Can you work these out from the model? Positions are in its coordinate system, mm. Coordinates: 2 decimals unless noted, no trailing zeros. Order: outer loops, then holes, each group sorted by start corner. A loop starts at its lowest first (then second) coordinate and runs counter-clockwise, first axis right, second up. Notation, with made-up numbers: (15, 6) -> (72, 6) arc R35 cw to (72, 45) -> close; hole circle Ø2 at (29, 71). An arc over 180 degrees is marked (long way). Answer as CSV lines item,"result".
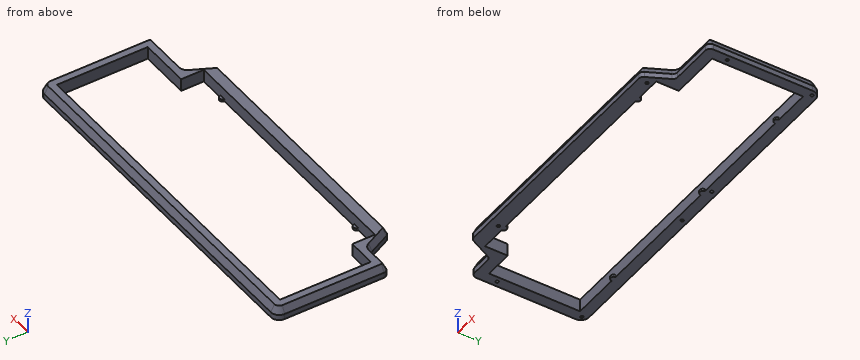
from build123d import *

# Parameters (mm, degrees)
PAD_DEPTH      = 10.6
PAD005_DEPTH   = 2
FILLET_R       = 4
FILLET014_R    = 7
CHAMFER_SIZE2  = 6
CHAMFER_SIZE   = 3
SKETCH020_R    = 1.25
HOLE007_DEPTH  = 5
HOLE007_TIPS_R = 1.25


with BuildPart() as part:
    # Sketch → Pad (new body)
    with BuildSketch(Plane.XY):
        Polygon((-152.075, 56.825), (152.075, 56.825), (152.075, -37.775), (109.7375, -37.775), (98.7125, -59.825), (-117.7625, -59.825), (-128.7875, -37.775), (-152.075, -37.775), align=None)
        Polygon((-143.075, 47.825), (143.075, 47.825), (143.075, -28.775), (100.2125, -28.775), (100.2125, -47.825), (-119.2625, -47.825), (-119.2625, -28.775), (-143.075, -28.775), align=None, mode=Mode.SUBTRACT)
    extrude(amount=PAD_DEPTH)

    # Sketch011 (on Face17 of Pad) → Pad005 (join)
    with BuildSketch(Plane(origin=(0, 0, 0), x_dir=(1, 0, 0), z_dir=(0, 0, -1))):
        with BuildLine():
            ThreePointArc((16.752533, -47.408333), (14.2875, -45.325), (11.822467, -47.408333))
            ThreePointArc((11.32946, -47.825), (11.652209, -47.706881), (11.822467, -47.408333))
            Line((11.32946, -47.825), (17.24554, -47.825))
            ThreePointArc((16.752533, -47.408333), (16.922791, -47.706881), (17.24554, -47.825))
        make_face()
        with BuildLine():
            ThreePointArc((112.002533, -47.408333), (109.5375, -45.325), (107.072467, -47.408333))
            ThreePointArc((106.57946, -47.825), (106.902209, -47.706881), (107.072467, -47.408333))
            Line((106.57946, -47.825), (112.49554, -47.825))
            ThreePointArc((112.002533, -47.408333), (112.172791, -47.706881), (112.49554, -47.825))
        make_face()
        with BuildLine():
            ThreePointArc((-97.547467, -47.408333), (-100.0125, -45.325), (-102.477533, -47.408333))
            ThreePointArc((-102.97054, -47.825), (-102.647791, -47.706881), (-102.477533, -47.408333))
            Line((-102.97054, -47.825), (-97.05446, -47.825))
            ThreePointArc((-97.547467, -47.408333), (-97.377209, -47.706881), (-97.05446, -47.825))
        make_face()
        with BuildLine():
            ThreePointArc((73.734967, 47.408333), (76.2, 45.325), (78.665033, 47.408333))
            ThreePointArc((79.15804, 47.825), (78.835291, 47.706881), (78.665033, 47.408333))
            Line((73.24196, 47.825), (79.15804, 47.825))
            ThreePointArc((73.734967, 47.408333), (73.564709, 47.706881), (73.24196, 47.825))
        make_face()
        with BuildLine():
            ThreePointArc((-97.715033, 47.408333), (-95.25, 45.325), (-92.784967, 47.408333))
            ThreePointArc((-92.29196, 47.825), (-92.614709, 47.706881), (-92.784967, 47.408333))
            Line((-98.20804, 47.825), (-92.29196, 47.825))
            ThreePointArc((-97.715033, 47.408333), (-97.885291, 47.706881), (-98.20804, 47.825))
        make_face()
    extrude(amount=-PAD005_DEPTH)

    # Fillet
    fillet_edges = [part.edges().sort_by_distance(p)[0] for p in [
        (98.7125, -59.825, 5.3),
        (109.7375, -37.775, 5.3),
        (152.075, -37.775, 5.3),
        (-117.7625, -59.825, 5.3),
        (-152.075, -37.775, 5.3),
        (-128.7875, -37.775, 5.3),
    ]]
    fillet(fillet_edges, radius=FILLET_R)

    # Fillet014
    fillet014_edges = [part.edges().sort_by_distance(p)[0] for p in [
        (152.075, 56.825, 5.3),
        (-152.075, 56.825, 5.3),
    ]]
    fillet(fillet014_edges, radius=FILLET014_R)

    # Chamfer
    chamfer_edges = [part.edges().sort_by_distance(p)[0] for p in [
        (-9.525, -59.825, 10.6),
    ]]
    chamfer_side = part.faces().sort_by_distance((148.817479, 8.025, 10.6))[0]
    chamfer(chamfer_edges, length=CHAMFER_SIZE, length2=CHAMFER_SIZE2, reference=chamfer_side)

    # Sketch020 (on Face4 of Chamfer) → Hole007 (cut)
    with BuildSketch(Plane(origin=(0, 0, 0), x_dir=(1, 0, 0), z_dir=(0, 0, -1))):
        with Locations((95.25, 52.325)):
            Circle(SKETCH020_R)
        with Locations((147.575, 19.05)):
            Circle(SKETCH020_R)
        with Locations((147.575, -52.325)):
            Circle(SKETCH020_R)
        with Locations((19.05, -52.325)):
            Circle(SKETCH020_R)
        with Locations((-19.05, -52.325)):
            Circle(SKETCH020_R)
        with Locations((-147.575, -52.325)):
            Circle(SKETCH020_R)
        with Locations((-147.575, 19.05)):
            Circle(SKETCH020_R)
        with Locations((-95.25, 52.325)):
            Circle(SKETCH020_R)
    extrude(amount=-HOLE007_DEPTH, mode=Mode.SUBTRACT)

    # Hole007 tips → Hole007 tip 1 section 0
    with BuildSketch(Plane(origin=(0, 0, 5), x_dir=(1, 0, 0), z_dir=(0, 0, -1)), mode=Mode.PRIVATE) as hole007_tip_1_s0:
        with Locations((95.25, 52.325)):
            Circle(HOLE007_TIPS_R)
    loft([hole007_tip_1_s0.sketch, Vertex(95.25, -52.325, 5.751076)], mode=Mode.SUBTRACT)

    # Hole007 tips → Hole007 tip 2 section 0
    with BuildSketch(Plane(origin=(0, 0, 5), x_dir=(1, 0, 0), z_dir=(0, 0, -1)), mode=Mode.PRIVATE) as hole007_tip_2_s0:
        with Locations((147.575, 19.05)):
            Circle(HOLE007_TIPS_R)
    loft([hole007_tip_2_s0.sketch, Vertex(147.575, -19.05, 5.751076)], mode=Mode.SUBTRACT)

    # Hole007 tips → Hole007 tip 3 section 0
    with BuildSketch(Plane(origin=(0, 0, 5), x_dir=(1, 0, 0), z_dir=(0, 0, -1)), mode=Mode.PRIVATE) as hole007_tip_3_s0:
        with Locations((147.575, -52.325)):
            Circle(HOLE007_TIPS_R)
    loft([hole007_tip_3_s0.sketch, Vertex(147.575, 52.325, 5.751076)], mode=Mode.SUBTRACT)

    # Hole007 tips → Hole007 tip 4 section 0
    with BuildSketch(Plane(origin=(0, 0, 5), x_dir=(1, 0, 0), z_dir=(0, 0, -1)), mode=Mode.PRIVATE) as hole007_tip_4_s0:
        with Locations((19.05, -52.325)):
            Circle(HOLE007_TIPS_R)
    loft([hole007_tip_4_s0.sketch, Vertex(19.05, 52.325, 5.751076)], mode=Mode.SUBTRACT)

    # Hole007 tips → Hole007 tip 5 section 0
    with BuildSketch(Plane(origin=(0, 0, 5), x_dir=(1, 0, 0), z_dir=(0, 0, -1)), mode=Mode.PRIVATE) as hole007_tip_5_s0:
        with Locations((-19.05, -52.325)):
            Circle(HOLE007_TIPS_R)
    loft([hole007_tip_5_s0.sketch, Vertex(-19.05, 52.325, 5.751076)], mode=Mode.SUBTRACT)

    # Hole007 tips → Hole007 tip 6 section 0
    with BuildSketch(Plane(origin=(0, 0, 5), x_dir=(1, 0, 0), z_dir=(0, 0, -1)), mode=Mode.PRIVATE) as hole007_tip_6_s0:
        with Locations((-147.575, -52.325)):
            Circle(HOLE007_TIPS_R)
    loft([hole007_tip_6_s0.sketch, Vertex(-147.575, 52.325, 5.751076)], mode=Mode.SUBTRACT)

    # Hole007 tips → Hole007 tip 7 section 0
    with BuildSketch(Plane(origin=(0, 0, 5), x_dir=(1, 0, 0), z_dir=(0, 0, -1)), mode=Mode.PRIVATE) as hole007_tip_7_s0:
        with Locations((-147.575, 19.05)):
            Circle(HOLE007_TIPS_R)
    loft([hole007_tip_7_s0.sketch, Vertex(-147.575, -19.05, 5.751076)], mode=Mode.SUBTRACT)

    # Hole007 tips → Hole007 tip 8 section 0
    with BuildSketch(Plane(origin=(0, 0, 5), x_dir=(1, 0, 0), z_dir=(0, 0, -1)), mode=Mode.PRIVATE) as hole007_tip_8_s0:
        with Locations((-95.25, 52.325)):
            Circle(HOLE007_TIPS_R)
    loft([hole007_tip_8_s0.sketch, Vertex(-95.25, -52.325, 5.751076)], mode=Mode.SUBTRACT)


solid = part.part
Q1. If I drill on line 1 (Y direction, x = 19.05, z = 3.75) (3 decimals); line 2 (X direction, y = -19.05, z = 3.8) (3 decimals); line 3 (X direction, y = -1, z = 2.25) (3 decimals), over which ranges is the centre line in solid material (lowest first)?
Solution:
line 1,"-59.825 to -47.825, 47.825 to 51.075, 53.575 to 56.825"
line 2,"-152.075 to -148.825, -146.325 to -143.075, 143.075 to 146.325, 148.825 to 152.075"
line 3,"-152.075 to -143.075, 143.075 to 152.075"
Q2. For P1, Ø2, axis at x = 19.05, y = 52.325, coming from the -Z side; P2, Ø0.8, axis at x = -100.5, y = 47, coming from the +Z side; P3, Ø2, axis at x = 9, z = 8, coming from the +Y side (3 decimals); P4, Ø5, axis at x = -67.5, y = -44.5, coming from the -Z side, each with a flat end and sliding along its axis, tell me the tip position at first contact or that it passes through.
Solution:
P1,"z = 5.15"
P2,"z = 2"
P3,"y = 55.625"
P4,"through"
Q3. Imagine slicing it at A-A (x = -5.5). List the corners of the cut face in (y, z) for me (3 decimals).
Solution:
outline,"(-59.825, 0) -> (-47.825, 0) -> (-47.825, 10.6) -> (-56.825, 10.6) -> (-59.825, 4.6) -> close; (47.825, 0) -> (56.825, 0) -> (56.825, 4.6) -> (53.825, 10.6) -> (47.825, 10.6) -> close"
